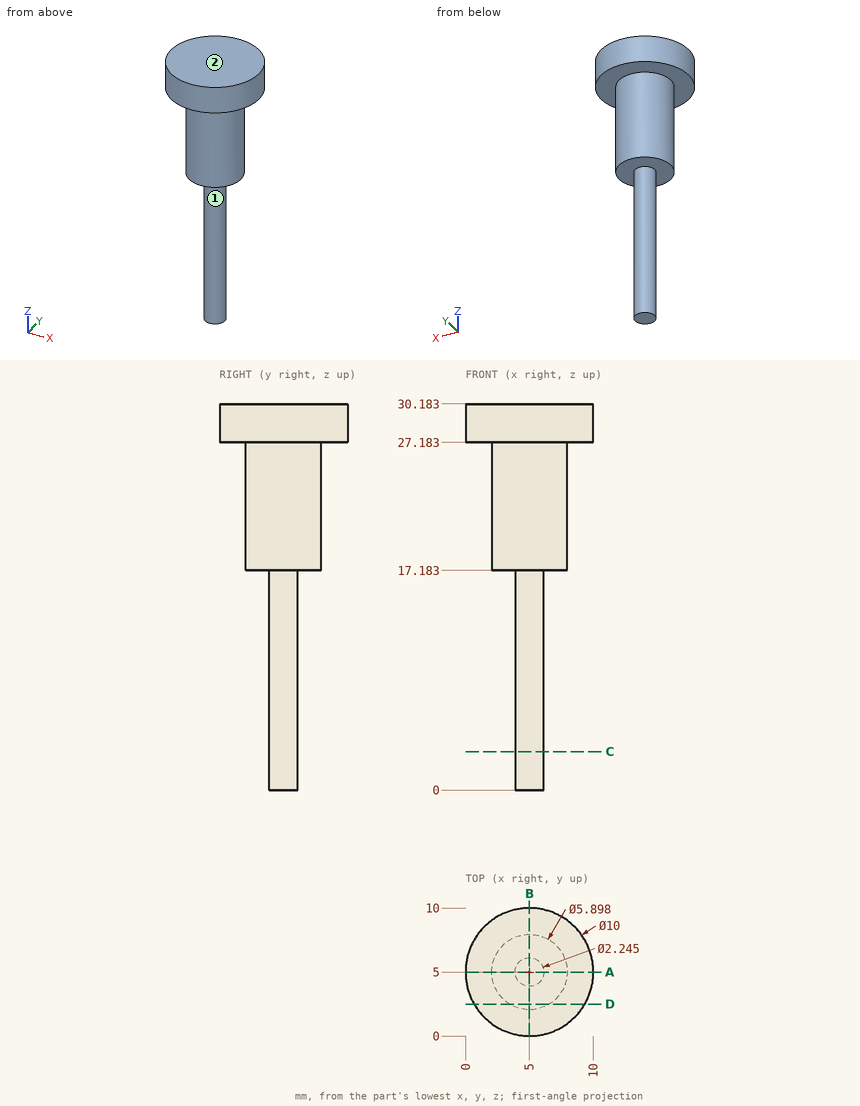
Geometry check sheet. Reference: drawing and pictorial views, mm from the part's lowest x, y, z. A direction names the side the tool comes from. Round coordinates to 2 decimals unless told otherwise and drop trailing zeros. Order: outer loops, then holes, each group sorted by start corner. A loop starts at its lowest first (then second) coordinate and runs counter-clockwise, first axis right, second up. Notation, with made-up numbers: M 44.5,24 L 75.5,24 A24 ccw 75.5,49 Z; hole C 68.25,54 d1. An arc over 180 degrees is marked long. One line per item, written item: value. Start each with the question number.
1. Scan lines: line 1 along Z through (x, y) = (8.5, 2.5); line 2 along Z through (x, y) = (3.75, 4.5); line 3 along Y through (x, z) = (5, 2). Record each from-to range of solid material in increasing order.
2. Access from +Z, -Z, +X, -X, +Y, -Y to the whole of each face (thin tool, end or side, straight path). Record for the marked faces 1 and 2.
3. Section check A-A on y = 5. Enter the section's corners in (x, z).
4. Section check C-C on z = 3. Enter the section's corners in (x, y) (1 decimal).
5. Section check D-D on y = 2.5. Enter the section's corners in (x, z).
6. Gauge pin test, flat ends, axial feed: P1, Ø1.5, axis at x = 2.5, z = 13, coming from the +Y side; P2, Ø3, axis at y = 7, z = 22, coming from the -X side. Record the tip position at first contact, or that the pin passes through.
Results found:
1. line 1: 27.18 to 30.18
1. line 2: 17.18 to 30.18
1. line 3: 3.88 to 6.12
2. face 1: -Z
2. face 2: +Z, +X, -X, +Y, -Y
3. outline: M 0,27.18 L 2.05,27.18 L 2.05,17.18 L 3.88,17.18 L 3.88,0 L 6.12,0 L 6.12,17.18 L 7.95,17.18 L 7.95,27.18 L 10,27.18 L 10,30.18 L 0,30.18 Z
4. outline: C 5,5 d2.2
5. outline: M 0.67,27.18 L 3.44,27.18 L 3.44,17.18 L 6.56,17.18 L 6.56,27.18 L 9.33,27.18 L 9.33,30.18 L 0.67,30.18 Z
6. P1: through
6. P2: x = 2.09
